Can you work these out from the model? Positions are in its coordinate system, mm. A direction names the side the tool comes from. Coordinates: 2 decimals unless noted, no trailing zeros. Order: outer loops, then holes, each group sorted by start corner. A loop starts at its lowest first (then second) coordinate and runs counter-clockwise, first axis right, second up. Notation, with made-up numbers: (-16.75, 25) -> (34.25, 25) arc R30 cw to (34.25, 63) -> close; hole circle Ø1 at (57, 74.5). An arc over 180 degrees is marked (long way). Return JSON: item names as keys, results as strings. Group by question number.
1) If we section it at B-B, the plane z = 3.6: Please give me the cut outline in (x, y) (3 decimals), then the cut area to 3 significant figures.
2) If we section it at C-C, the plane y = 53: Please give me the cut outline in (x, z).
3) If I drill on probe 1 along Y at (x, z) = (-27.5, 1.05) (3 decimals); probe 2 along X at (y, z) = (9.5, 2.8), over which ranges is the centre line in solid material (lowest first)? Write a range as from..to.
4) For pin 1 (2 mm diameter, centred on y = -7.5, z = 3.5, fed in from +X); pin 2 (1.8 mm diameter, centred on y = -50, z = 1.5, fed in from -X), each with a flat end and sliding along its axis, tell me the tip position at first contact or that it passes through.
5) If we section it at A-A, the plane x = -25: Please give me the cut outline in (y, z) (3 decimals).
6) Thinking about a two-plate mould opening in Y: for faces 1 (the flat face through (-42, 1, 0)), 2 (the flat face through (-26, 12.375, 3)), which applies, +Y half, -Y half, draft (parallel to the pull), parting line (faces both ways), or undercut?
7) For faces 3 (the flat face through (-57, -37.125, 3)), 4 (the flat face through (-26, -12.375, 3)), 5 (the flat face through (-23, -25, 3)), which set-ups out of +Z, -Z, +X, -X, +Y, -Y let a thin tool reach every point of the face, with its end or its side?
Autodesk Inventor part; units mm, degrees
ref_plane "YZ Plane" through (0, 0, 0) normal (1, 0, 0) x (0, 1, 0)
ref_plane "XZ Plane" through (0, 0, 0) normal (0, 1, 0) x (-1, 0, 0)
ref_plane "XY Plane" through (0, 0, 0) normal (0, 0, 1) x (1, 0, 0)
sketch "Sketch1" plane through (0, 0, 0) normal (0, 0, 1) x (1, 0, 0)
  line L0 (-23, -100) -> (-60, -100)
  line L1 (-60, -100) -> (-60, 100)
  line L2 (-60, 100) -> (-23, 100)
  line L3 (-23, 100) -> (-23, -100)
  line L4 (-23, -100) -> (-60, 100) construction
  line L5 (-60, -100) -> (-23, 100) construction
  line L6 (-23, 0) -> (-23, 12.375)
  line L7 (-23, 12.375) -> (-29, 12.375)
  line L8 (-29, 12.375) -> (-29, -12.375)
  line L9 (-29, -12.375) -> (-23, -12.375)
  line L10 (-23, 12.375) -> (-23, 37.125)
  line L11 (-23, 37.125) -> (-29, 37.125)
  line L12 (-29, 37.125) -> (-29, 61.875)
  line L13 (-29, 61.875) -> (-23, 61.875)
  line L14 (-23, -12.375) -> (-23, -37.125)
  line L15 (-23, -37.125) -> (-29, -37.125)
  line L16 (-29, -37.125) -> (-29, -61.875)
  line L17 (-29, -61.875) -> (-23, -61.875)
  line L18 (-41.5, 0) -> (-41.5, 100)
  line L19 (-41.5, 0) -> (-25.6792, 0)
  line L20 (-60, 12.375) -> (-54, 12.375)
  line L21 (-54, 12.375) -> (-54, -12.375)
  line L22 (-54, -12.375) -> (-60, -12.375)
  line L23 (-60, 37.125) -> (-54, 37.125)
  line L24 (-54, 37.125) -> (-54, 61.875)
  line L25 (-54, 61.875) -> (-60, 61.875)
  line L26 (-60, -37.125) -> (-54, -37.125)
  line L27 (-54, -37.125) -> (-54, -61.875)
  line L28 (-54, -61.875) -> (-60, -61.875)
  dimension "d18" = 37
  dimension "d19" = 200
  dimension "d20" = 12.375
  dimension "d21" = 6
  dimension "d22" = 24.75
  dimension "d23" = 24.75
  dimension "d24" = 6
  dimension "d25" = 24.75
  dimension "d26" = 24.75
  dimension "d27" = 6
  dimension "d28" = 24.75
extrude "Extrusion1" add sketch "Sketch1" along normal blind 6 contours L0 L1 L28 L27 L26 L22 L21 L20 L23 L24 L25 L2 L18 L19 L8 L9 L3 L15 L16 L17 | L7 L8 L19 L18 L2 L3 L13 L12 L11
properties part number "Frontandback_2"
Result sheet:
{
 "1": {"outline": "(-60, -100) -> (-23, -100) -> (-23, -61.875) -> (-29, -61.875) -> (-29, -37.125) -> (-23, -37.125) -> (-23, -12.375) -> (-29, -12.375) -> (-29, 12.375) -> (-23, 12.375) -> (-23, 37.125) -> (-29, 37.125) -> (-29, 61.875) -> (-23, 61.875) -> (-23, 100) -> (-60, 100) -> (-60, 61.875) -> (-54, 61.875) -> (-54, 37.125) -> (-60, 37.125) -> (-60, 12.375) -> (-54, 12.375) -> (-54, -12.375) -> (-60, -12.375) -> (-60, -37.125) -> (-54, -37.125) -> (-54, -61.875) -> (-60, -61.875) -> close", "area": "6,510 mm2"},
 "2": {"outline": "(-54, 0) -> (-29, 0) -> (-29, 6) -> (-54, 6) -> close"},
 "3": {"probe 1": "y = -100..-61.875, -37.125..-12.375, 12.375..37.125, 61.875..100", "probe 2": "x = -54..-29"},
 "4": {"pin 1": "stops at x = -29", "pin 2": "stops at x = -54"},
 "5": {"outline": "(-100, 0) -> (-61.875, 0) -> (-61.875, 6) -> (-100, 6) -> close; (-37.125, 0) -> (-12.375, 0) -> (-12.375, 6) -> (-37.125, 6) -> close; (12.375, 0) -> (37.125, 0) -> (37.125, 6) -> (12.375, 6) -> close; (61.875, 0) -> (100, 0) -> (100, 6) -> (61.875, 6) -> close"},
 "6": {"face 1": "draft", "face 2": "undercut"},
 "7": {"face 3": "+Z, -Z, -X", "face 4": "+Z, -Z, +X", "face 5": "+Z, -Z, +X, +Y, -Y"}
}
